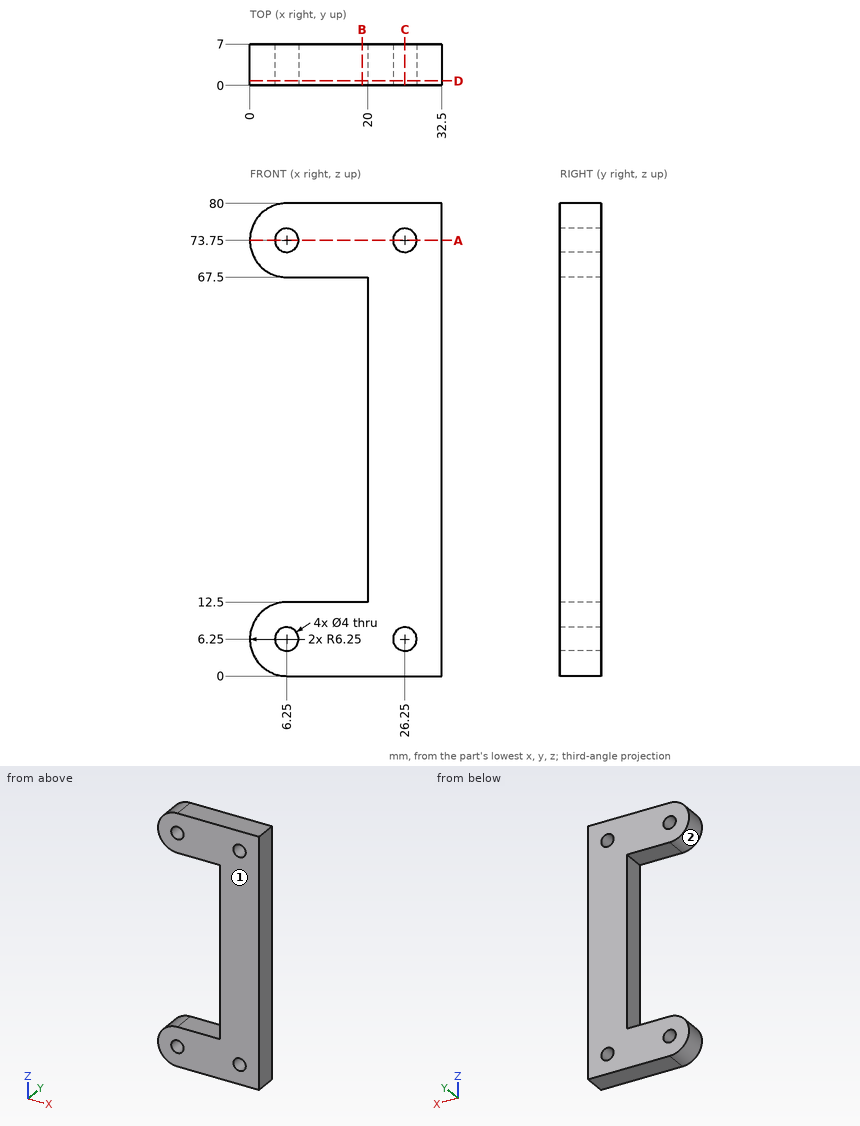
Answer from the drawing. Dimensions are ordinates in mm from the lowest x, y and z of the part. Give positions to 0.01 mm unless a question says otherwise; leave off trailing zeros. Write each loop counter-clockwise with the first axis right and the second up, starting at its lowest first coordinate (ties: lowest second). Pieces come first, ordered by that corner, then holes. Notation, with made-up numbers: (-17, 76.25) -> (35, 76.25) arc R22 cw to (35, 104.25) -> close; hole circle Ø9 at (-1, 59). An arc over 180 degrees is marked (long way). Use a Markdown table: item, result.
(1) Flat-ended cylindrical pins translate along their axes: P1, Ø3, axis at y = 1, z = 24, coming from the -X side; P2, Ø4, axis at y = 3, z = 12, coming from the -X side; P3, Ø1, axis at x = 18, z = 35.5, coming from the +Y side. Find the tip coordinate at first contact, or state that the pin passes through.
Return value:
| item | result |
|---|---|
| P1 | x = 20 |
| P2 | x = 1.25 |
| P3 | through |
(2) Section A-A, the plane z = 73.75 is taken. Determine the outline of the cut face in (x, y), then the cut area to 4 significant figures.
Return value:
| item | result |
|---|---|
| outline | (0, 0) -> (4.25, 0) -> (4.25, 7) -> (0, 7) -> close; (8.25, 0) -> (24.25, 0) -> (24.25, 7) -> (8.25, 7) -> close; (28.25, 0) -> (32.5, 0) -> (32.5, 7) -> (28.25, 7) -> close |
| area | 171.5 mm2 |
(3) Determine the mould class of the marked faces 1 and 2 for opening direction Z: released by +Z, released by -Z, zero draft, split by the parting line, or undercut.
Return value:
| item | result |
|---|---|
| face 1 | zero draft |
| face 2 | undercut |
(4) Find the intervals of material crossed by probe 1 along X at (y, z) = (3.25, 73.75); probe 2 along Z at (x, y) = (26.25, 3.75); probe 3 along Z at (x, y) = (18, 0.75), in increasing order. Write a range as from..to.
Return value:
| item | result |
|---|---|
| probe 1 | 0..4.25, 8.25..24.25, 28.25..32.5 |
| probe 2 | 0..4.25, 8.25..71.75, 75.75..80 |
| probe 3 | 0..12.5, 67.5..80 |
(5) Section B-B, the plane x = 19 is taken. Determine the outline of the cut face in (y, z).
Return value:
| item | result |
|---|---|
| outline | (0, 0) -> (7, 0) -> (7, 12.5) -> (0, 12.5) -> close; (0, 67.5) -> (7, 67.5) -> (7, 80) -> (0, 80) -> close |
(6) Section C-C, the plane x = 26.25 is taken. Determine the outline of the cut face in (y, z), then the cut area to 3 significant figures.
Return value:
| item | result |
|---|---|
| outline | (0, 0) -> (7, 0) -> (7, 4.25) -> (0, 4.25) -> close; (0, 8.25) -> (7, 8.25) -> (7, 71.75) -> (0, 71.75) -> close; (0, 75.75) -> (7, 75.75) -> (7, 80) -> (0, 80) -> close |
| area | 504 mm2 |
(7) Section D-D, the plane y = 0.75 is taken. Determine the outline of the cut face in (x, z).
Return value:
| item | result |
|---|---|
| outline | (6.25, 0) -> (32.5, 0) -> (32.5, 80) -> (6.25, 80) arc R6.25 ccw to (6.25, 67.5) -> (20, 67.5) -> (20, 12.5) -> (6.25, 12.5) arc R6.25 ccw to start; hole circle Ø4 at (6.25, 6.25); hole circle Ø4 at (6.25, 73.75); hole circle Ø4 at (26.25, 6.25); hole circle Ø4 at (26.25, 73.75) |
